Input: part model. Units: mm. Frame: model coordinates. A direction names the side the tool comes from. Coordinates: 2 decimals unless noted, no trailing zeros. Write each loop counter-clockwise with the first axis right and the second up, starting at its lowest first coordinate (ties: lowest second). Pieces come first, ordered by that corner, then holes. Notation, with made-up numbers: (85.5, 21.5) - (115.5, 21.5) arc R11 cw to (115.5, 33.5) - close; hole circle Ø2 at (35, 5). An arc over 180 degrees is marked (long way). Use a Markdown table: item, result. Add a question column.
Q1. Pin query (flat end, axial travel): P1, Ø0.7, axis at y = 0.5, z = 1.5, coming from the -X side; P2, Ø8, axis at x = -7, z = 0.5, coming from the -Y side; P3, Ø1, axis at x = -7.5, y = 2, coming from the -Z side. Return the tip coordinate at first contact, or that it passes through.
Q2. Section query C-C (z = -4.5). Return the cut outline in (x, y), then the cut area to 3 significant figures.
Q3. Material intervals for probe 1 along Z at (x, y) = (4, 0.7); probe 2 along Z at (x, y) = (-4.25, 0.2); probe 3 along Y at (x, z) = (-3, -9.25), sorted ascending. Write a range as from..to.
Q4. Section query B-B (y = 0.7). Return the cut outline in (x, z), then the cut area to 3 significant figures.
Q5. Section query D-D (x = -0.75). Return the cut outline in (y, z).
Q6. Mould query, pull axis Z, two halves, no side actions, for faces 4 (the face through (5.66, 0.59, -0.37)), 5 (the face through (10, 0.5, -0.1)), 6 (the face through (-1.13, 2.4, 10.93)). Classes: released by +Z, released by -Z, zero draft, split by the parting line, or undercut.
Q7. Set-up query: faces 1 (the face through (-5, 1, -10.1)), 2 (the face through (9.43, 2.4, 0.13)), 3 (the face through (1.026, 2.746, -0.391)). Return all of +Z, -Z, +X, -X, +Y, -Y with unobstructed straight access to the full face (end or side cutting, diameter ignored); none if empty.
Autodesk Inventor part; units mm, degrees
ref_plane "YZ Plane" through (0, 0, 0) normal (1, 0, 0) x (0, 1, 0)
ref_plane "XZ Plane" through (0, 0, 0) normal (0, 1, 0) x (-1, 0, 0)
ref_plane "XY Plane" through (0, 0, 0) normal (0, 0, 1) x (1, 0, 0)
sketch "Sketch1" plane through (0, 0, 0) normal (0, 1, 0) x (-1, 0, 0)
  line L0 (-10, 11.5) -> (10, 11.5)
  line L1 (10, 11.5) -> (10, -11.5)
  line L2 (10, -11.5) -> (-10, -11.5)
  line L3 (-10, -11.5) -> (-10, 11.5)
  line L4 (-10, 11.5) -> (10, -11.5) construction
  line L5 (10, 11.5) -> (-10, -11.5) construction
  point P0 (0, 0)
  dimension "d0" = 20
  dimension "d1" = 23
extrude "Extrusion1" add sketch "Sketch1" along normal blind 3
sketch "Sketch2" plane through (0, 0, 0) normal (0, -1, 0) x (1, 0, 0)
  line L0 (10, -11.5) -> (-10, -11.5)
  line L1 (10, 11.5) -> (10, -11.5)
  line L2 (-10, 11.5) -> (10, 11.5)
  line L3 (-10, -11.5) -> (-10, 11.5)
  line L4 (0, -10.1) -> (-10, -10.1)
  line L5 (-10, -10.1) -> (-10, 10.1)
  line L6 (-10, 10.1) -> (0, 10.1)
  line L7 (0, 10.1) -> (0, -10.1)
  line L8 (0, -10.1) -> (-10, 10.1) construction
  line L9 (-10, -10.1) -> (0, 10.1) construction
  line L10 (-10, -11.5) -> (-10, 11.5)
  point P0 (0, 0)
  point P1 (-5, 0)
  dimension "d4" = 20.2
  dimension "d5" = 10
extrude "Extrusion2" cut sketch "Sketch2" against normal blind 1.4 contours L3 L6 L7 L4
sketch "Sketch3" plane through (0, 3, 0) normal (0, 1, 0) x (1, 0, 0)
  line L0 (10, -11.5) -> (10, 11.5)
  point P0 (0, 0)
  point P1 (4, 0)
  dimension "d8" = 6
hole "Hole1" at (4, 3, 0) direction (0, -1, 0) diameter 3.4 end through all counterbore diameter 6 counterbore depth 0.5
chamfer "Chamfer1" distance 1.3 angle 45 1 edges at (4, 2.5, -1.7)
fillet "Fillet1" radius 2 3 edges at (0, 3, 11.5) (10, 3, 0) (0, 3, -11.5)
fillet "Fillet2" radius 2 4 edges at (9.4142, 2.4142, 10.9142) (10, 0.5, 11.5) (9.4142, 2.4142, -10.9142) (10, 0.5, -11.5)
properties part number "LIKA LKM-1439"
Values follow:
| question | item | result |
|---|---|---|
| 1 | P1 | x = 0 |
| 1 | P2 | y = 1.4 |
| 1 | P3 | z = -11.44 |
| 2 | outline | (-10, 1.4) - (0, 1.4) - (0, 0) - (10, 0) - (10, 1) arc R2 ccw to (8, 3) - (-10, 3) - close |
| 2 | area | 45.1 mm2 |
| 3 | probe 1 | -11.5..-1.7, 1.7..11.5 |
| 3 | probe 2 | -11.5..-10.1, 10.1..11.5 |
| 3 | probe 3 | 1.4..3 |
| 4 | outline | (-10, -11.5) - (8, -11.5) arc R2 ccw to (10, -9.5) - (10, 9.5) arc R2 ccw to (8, 11.5) - (-10, 11.5) - (-10, 10.1) - (0, 10.1) - (0, -10.1) - (-10, -10.1) - close; hole circle Ø3.4 at (4, 0) |
| 4 | area | 247 mm2 |
| 5 | outline | (0, -11.5) - (1, -11.5) arc R2 ccw to (3, -9.5) - (3, 9.5) arc R2 ccw to (1, 11.5) - (0, 11.5) - (0, 10.1) - (1.4, 10.1) - (1.4, -10.1) - (0, -10.1) - close |
| 6 | face 4 | undercut |
| 6 | face 5 | zero draft |
| 6 | face 6 | released by +Z |
| 7 | face 1 | -X, -Y |
| 7 | face 2 | +Z, -Z, +X, +Y |
| 7 | face 3 | +Y |
